Verification items for the finished model (mm, model axes). Face numbers are marked on the shaded views. A direction names the side the tool comes from. Round coordinates to 2 decimals unless told otherwise and drop trailing zeros. Write each loop counter-clockwise with the first axis right and the second up, starting at its lowest first coordinate (ties: lowest second). Pieces come first, ordered by that corner, then holes. Notation, with made-up numbers: M 77,70 L 96,70 A15 ccw 96,78 Z; hole C 77,51.25 d5. An arc over 180 degrees is marked long. One line per item, written item: value. Start each with the question number.
Item 1: Thickness scan on probe 1 along Y at (x, z) = (39, 11.5); probe 2 along Y at (x, z) = (29.5, 18.5); probe 3 along Z at (x, y) = (-22, -12). Record the ranges inside material, lowest first. Write a range as from..to.
Item 2: Tool access check on the marked faces 1 and 2. Record the directions out of +Z, -Z, +X, -X, +Y, -Y that give a thin tool (end or side, any length) a straight path to the whole face; none if there is none.
Item 3: Section check C-C, the plane y = 12. Record the cut outline in (x, z).
Item 4: Section check B-B, the plane x = -17. Record the cut outline in (y, z).
Item 5: Section check A-A, the plane z = 15. Record the cut outline in (x, y).
Item 6: Gauge pin test, flat ends, axial feed: pin 1 (8 mm diameter, centred on x = -27.5, z = 16.5, fed in from +Y); pin 2 (10 mm diameter, centred on x = 37, z = 13, fed in from -Y); pin 3 (6 mm diameter, centred on y = -6.5, z = 15, fed in from -X); pin 4 (4 mm diameter, centred on y = 6, z = 17, fed in from +X). Record the tip position at first contact, or that the pin passes through.
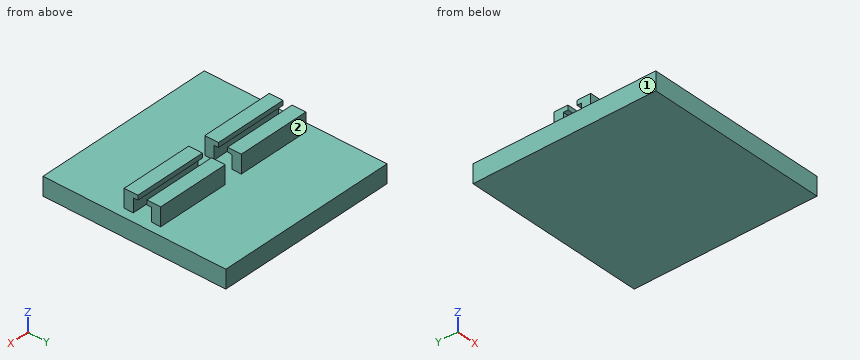
from build123d import *

# Parameters (mm, degrees)
SKETCH1_W               = 100
SKETCH1_H               = 100
BACK_PLATE_DEPTH        = 10
SKETCH2_W               = 40
SKETCH2_H               = 20
SLIDER_MOUNT_BOSS_DEPTH = 10
SLIDER_MOUNT_DEPTH      = 77.974021592


with BuildPart() as part:
    # Sketch1 → back plate (new body)
    with BuildSketch(Plane.XY):
        Rectangle(SKETCH1_W, SKETCH1_H)
    extrude(amount=BACK_PLATE_DEPTH)

    # Sketch2 → slider mount boss (add)
    with BuildSketch(Plane.XY.offset(10)):
        with Locations((-25, 0)):
            Rectangle(SKETCH2_W, SKETCH2_H)
    slider_mount_boss = extrude(amount=SLIDER_MOUNT_BOSS_DEPTH)

    # Sketch3 → slider mount (cut, through all)
    with BuildSketch(Plane(origin=(-5, 0, 0), x_dir=(0, 0, -1), z_dir=(1, 0, 0))):
        Polygon((-17.5, 5), (-10, 5), (-10, -5), (-17.5, -5), (-17.5, -2.5), (-20, -2.5), (-20, 2.5), (-17.5, 2.5), align=None)
    slider_mount = extrude(amount=-SLIDER_MOUNT_DEPTH, mode=Mode.SUBTRACT)

    # Mirror3: slider mount boss, slider mount across plane
    add(slider_mount_boss.mirror(Plane(origin=(0, 0, 0), x_dir=(0, 0, 1), z_dir=(1, 0, 0))))
    add(slider_mount.mirror(Plane(origin=(0, 0, 0), x_dir=(0, 0, 1), z_dir=(1, 0, 0))), mode=Mode.SUBTRACT)


solid = part.part
Response values:
1. probe 1: y = -10..-5, 5..10
1. probe 2: y = -10..-2.5, 2.5..10
1. probe 3: z = 0..10
2. face 1: +Z, -Z, -X, +Y, -Y
2. face 2: +Z, +X, -X, +Y
3. outline: M -50,0 L 50,0 L 50,10 L -50,10 Z
4. outline: M -50,0 L 50,0 L 50,10 L 10,10 L 10,20 L 2.5,20 L 2.5,17.5 L 5,17.5 L 5,10 L -5,10 L -5,17.5 L -2.5,17.5 L -2.5,20 L -10,20 L -10,10 L -50,10 Z
5. outline: M -45,-10 L -5,-10 L -5,-5 L -45,-5 Z; M -45,5 L -5,5 L -5,10 L -45,10 Z; M 5,-10 L 45,-10 L 45,-5 L 5,-5 Z; M 5,5 L 45,5 L 45,10 L 5,10 Z
6. pin 1: stops at y = 10
6. pin 2: stops at y = -50
6. pin 3: stops at x = -45
6. pin 4: stops at x = 45
